Design review of the part shown in the three views and the two pictorial views. Dimensions are in mm from the part's minimum x, y and z. A direction names the side the tool comes from. Round coordinates to 2 decimals unless told otherwise and drop trailing zeros. Write each loop counter-clockwise with the first axis right and the second up, starting at its lowest first coordinate (ties: lowest second). Pieces come first, ordered by that corner, then holes. Notation, with made-up numbers: (-10, 5.25) -> (39, 5.25) arc R16 cw to (39, 34.25) -> close; hole circle Ø11 at (54, 47.5). An arc over 180 degrees is marked (long way). Answer as a JSON object with one key per item and string values. Group by question number.
1) We need section D-D, the plane z = 33. Write out the cut boundary in (x, y).
2) Insertion check: pin 1 Ø2 at (y, z) = (23, 32.5) entering from -X; pin 2 Ø6 at (x, y) = (43, 85) entering from -Z. Each pin has a flat end and moves straight along its axis. Give the tip position at first contact, or say it passes through.
3) We need section A-A, the plane z = 76. Write out the cut boundary in (x, y), then the cut area to 3 significant figures.
4) We need section B-B, the plane y = 85. Write out the cut boundary in (x, z).
5) Machinability: for the marked faces 1 and 2, which of the approach directions +Z, -Z, +X, -X, +Y, -Y give a long, thin tool a straight path to every point of the face, cutting with its end or side? Answer none if there is none.
6) We need section C-C, the plane x = 127. Write out the cut boundary in (y, z).
7) To check wall thickness, follow probe 1 along Y at (x, z) = (127, 38); probe 2 along X at (y, z) = (76, 53); probe 3 along X at (y, z) = (17, 13). State the ranges of each line that lie inside material, in increasing order. Write a range as [from, to].
8) Mouldability with a two-part tool opening along Y and no side actions: class the marked faces 3, 4, 5 and 6 as pulls with the +Y half, pulls with the -Y half, needs draft (parallel to the pull), parting line crosses it, or undercut.
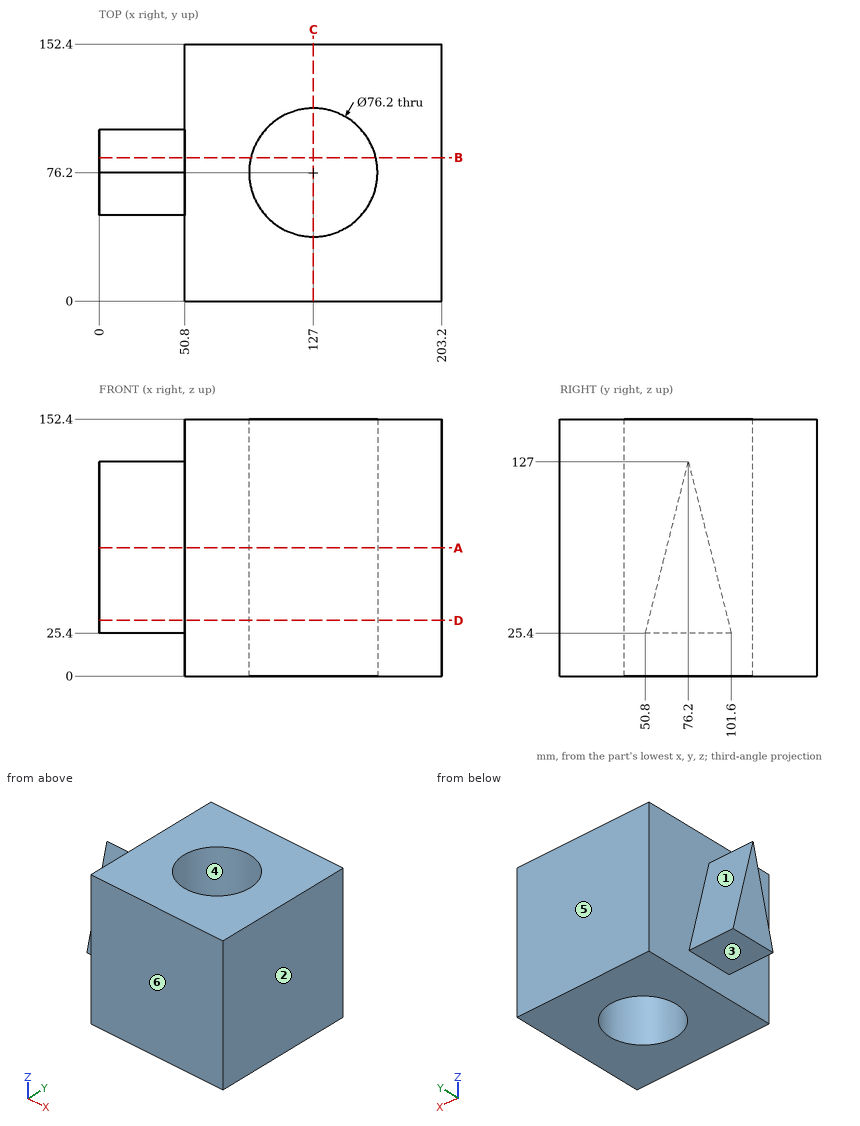
Here are the results:
{
 "1": {"outline": "(0, 52.7) -> (50.8, 52.7) -> (50.8, 0) -> (203.2, 0) -> (203.2, 152.4) -> (50.8, 152.4) -> (50.8, 99.7) -> (0, 99.7) -> close; hole circle Ø76.2 at (127, 76.2)"},
 "2": {"pin 1": "stops at x = 50.8", "pin 2": "stops at z = 25.4"},
 "3": {"outline": "(0, 63.45) -> (50.8, 63.45) -> (50.8, 0) -> (203.2, 0) -> (203.2, 152.4) -> (50.8, 152.4) -> (50.8, 88.95) -> (0, 88.95) -> close; hole circle Ø76.2 at (127, 76.2)", "area": "20,000 mm^2"},
 "4": {"outline": "(0, 25.4) -> (50.8, 25.4) -> (50.8, 0) -> (89.93, 0) -> (89.93, 152.4) -> (50.8, 152.4) -> (50.8, 91.8) -> (0, 91.8) -> close; (164.07, 0) -> (203.2, 0) -> (203.2, 152.4) -> (164.07, 152.4) -> close"},
 "5": {"face 1": "+Z, -X, +Y", "face 2": "+Z, -Z, +X, +Y, -Y"},
 "6": {"outline": "(0, 0) -> (38.1, 0) -> (38.1, 152.4) -> (0, 152.4) -> close; (114.3, 0) -> (152.4, 0) -> (152.4, 152.4) -> (114.3, 152.4) -> close"},
 "7": {"probe 1": "y = [0, 38.1], [114.3, 152.4]", "probe 2": "x = [0, 88.9], [165.1, 203.2]", "probe 3": "x = [50.8, 203.2]"},
 "8": {"face 3": "needs draft", "face 4": "undercut", "face 5": "pulls with the +Y half", "face 6": "pulls with the -Y half"}
}
